```python
from build123d import *

# Parameters (mm, degrees)
F0_W     = 39.6748
F0_H     = 39.6748
F0_R     = 17.4625
F0_R_2   = 16.8275
F1_DEPTH = 3.2004
F2_DEPTH = 20.066
F3_R     = 13.97
F4_DEPTH = 16.8656
F5_R     = 15.5
F6_DEPTH = 8.1026


with BuildPart() as f1:
    # F0 (on Front) → F1 (new body)
    with BuildSketch(Plane.XZ):
        Rectangle(F0_W, F0_H)
        with BuildLine():
            Line((-13.265674, -15.564284), (-14.252556, -16.518023))
            ThreePointArc((-14.252556, -16.518023), (-16.635155, -16.817997), (-16.716767, -14.417977))
            Line((-16.716767, -14.417977), (-15.697317, -13.421976))
            ThreePointArc((-15.697317, -13.421976), (-13.320738, -13.175603), (-13.265674, -15.564284))
        make_face(mode=Mode.SUBTRACT)
        with BuildLine():
            ThreePointArc((13.323525, -15.493634), (13.405137, -13.093613), (15.787736, -13.393587))
            Line((15.787736, -13.393587), (16.774618, -14.347326))
            ThreePointArc((16.774618, -14.347326), (16.719554, -16.736007), (14.342975, -16.489634))
            Line((14.342975, -16.489634), (13.323525, -15.493634))
        make_face(mode=Mode.SUBTRACT)
        with BuildLine():
            ThreePointArc((-16.716767, 14.417977), (-16.635155, 16.817997), (-14.252556, 16.518023))
            Line((-14.252556, 16.518023), (-13.265674, 15.564284))
            ThreePointArc((-13.265674, 15.564284), (-13.320738, 13.175603), (-15.697317, 13.421976))
            Line((-15.697317, 13.421976), (-16.716767, 14.417977))
        make_face(mode=Mode.SUBTRACT)
        Circle(F0_R, mode=Mode.SUBTRACT)
        with BuildLine():
            Line((16.774618, 14.347326), (15.787736, 13.393587))
            ThreePointArc((15.787736, 13.393587), (13.405137, 13.093613), (13.323525, 15.493634))
            Line((13.323525, 15.493634), (14.342975, 16.489634))
            ThreePointArc((14.342975, 16.489634), (16.719554, 16.736007), (16.774618, 14.347326))
        make_face(mode=Mode.SUBTRACT)
        Circle(F0_R)
        Circle(F0_R_2, mode=Mode.SUBTRACT)
        Circle(F0_R_2)
    extrude(amount=F1_DEPTH)

    # F0 (on Front) → F2 (join)
    with BuildSketch(Plane.XZ):
        Circle(F0_R)
        Circle(F0_R_2, mode=Mode.SUBTRACT)
    extrude(amount=F2_DEPTH)

    # F3 (on face) → F4 (join)
    with BuildSketch(Plane.XZ.offset(3.2004)):
        with BuildLine():
            ThreePointArc((1.5875, -15.157092), (11.323672, -10.19961), (15.24, 0))
            ThreePointArc((15.24, 0), (-10.19961, 11.323672), (-1.5875, -15.157092))
            Line((-1.5875, -15.157092), (1.5875, -15.157092))
        make_face()
        Circle(F3_R, mode=Mode.SUBTRACT)
        with BuildLine():
            ThreePointArc((1.5875, -15.157092), (0, -15.24), (-1.5875, -15.157092))
            Line((-1.5875, -15.157092), (-1.5875, -16.427092))
            Line((-1.5875, -16.427092), (1.5875, -16.427092))
            Line((1.5875, -16.427092), (1.5875, -15.157092))
        make_face()
        with BuildLine():
            Line((1.5875, -15.157092), (-1.5875, -15.157092))
            ThreePointArc((-1.5875, -15.157092), (0, -15.24), (1.5875, -15.157092))
        make_face()
    extrude(amount=F4_DEPTH)

    # F5 (on face) → F6 (join)
    with BuildSketch(Plane(origin=(0, 0, 0), x_dir=(-1, 0, 0), z_dir=(0, 1, 0))):
        Circle(F5_R)
    extrude(amount=F6_DEPTH)


solid = f1.part
```
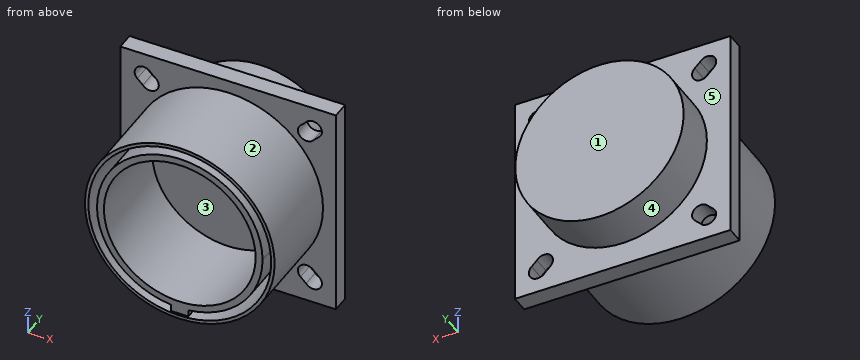
The listing builds one solid part. Answer for the finished solid, in the listing's coordinates (mm). Face numbers are marked on the shaded views. A direction names the side the tool comes from. Give positions to 0.01 mm unless a question says otherwise; leave off trailing zeros. Order: outer loops, then holes, each group sorted by start corner. A loop starts at its lowest first (then second) coordinate and runs counter-clockwise, first axis right, second up. Notation, with made-up numbers: M 25.25,81.25 L 45.25,81.25 A18 ccw 45.25,105.25 Z; hole C 73.25,41 d9. An arc over 180 degrees is marked long. Put each result on its own line as item: value. Start each with the question number.
Item 1: Which of the six approach directions +Z, -Z, +X, -X, +Y, -Y give full straight-line access (tool end or side, diameter ignored) to the marked faces 1 and 2?
Item 2: Find the intervals of material crossed by line 1 along X through (y, z) = (-6.75, -0.5); line 2 along X through (y, z) = (-1.75, -14.5); line 3 along X through (y, z) = (-6, -6.5), in increasing order.
Item 3: The part is cut by section C-C, the plane z = 6.5. Determine the outline of the cut face in (x, y), and give its area (3 significant figures).
Item 4: The part is cut by section B-B, the plane x = 8. Determine the outline of the cut face in (y, z), and give its area (3 significant figures).
Item 5: For a pull along X with two mould halves and no side action, classify the marked faces 3, 4 and 5 as +X half, -X half, draft (parallel to the pull), parting line (faces both ways), or undercut.
Item 6: The part is cut by section A-A, the plane y = -6. Determine the outline of the cut face in (x, z) (1 decimal), and give its area (3 significant figures).
Item 7: Flat-ended cylindrical pins translate along their axes: P1, Ø1, axis at y = -13.5, z = -16, coming from the -X side; P2, Ø2, axis at y = -13, z = 7.5, coming from the -X side; P3, Ø3, axis at x = 12, y = -8, coming from the -Z side. Find the tip coordinate at first contact, or state that the pin passes through.
Answer key:
1. face 1: +Z, -Z, +X, -X, +Y
1. face 2: -Y
2. line 1: x = -17.46 to -16.82, -15.23 to -13.96, 13.96 to 15.23, 16.82 to 17.46
2. line 2: x = -19.84 to -16.8, -12.77 to 12.84, 16.91 to 19.84
2. line 3: x = -16.21 to -15.52, -13.78 to -12.37, 12.37 to 13.78, 15.52 to 16.21
3. outline: M -19.84,-3.2 L -16.21,-3.2 L -16.21,-20.07 L -15.52,-20.07 L -15.52,-3.2 L -13.78,-3.2 L -13.78,-20.07 L -12.37,-20.07 L -12.37,-3.2 L 12.37,-3.2 L 12.37,-20.07 L 13.78,-20.07 L 13.78,-3.2 L 15.52,-3.2 L 15.52,-20.07 L 16.21,-20.07 L 16.21,-3.2 L 19.84,-3.2 L 19.84,0 L 14.07,0 L 14.07,8.1 L -14.07,8.1 L -14.07,0 L -19.84,0 Z
3. area: 426 mm²
4. outline: M -20.07,-15.52 L -3.2,-15.52 L -3.2,-19.84 L 0,-19.84 L 0,-13.28 L 8.1,-13.28 L 8.1,13.28 L 0,13.28 L 0,19.84 L -3.2,19.84 L -3.2,15.52 L -20.07,15.52 L -20.07,14.8 L -3.2,14.8 L -3.2,12.97 L -20.07,12.97 L -20.07,11.45 L -3.2,11.45 L -3.2,-11.45 L -20.07,-11.45 L -20.07,-12.97 L -3.2,-12.97 L -3.2,-14.8 L -20.07,-14.8 Z
4. area: 418 mm²
5. face 3: undercut
5. face 4: parting line
5. face 5: draft
6. outline: C 0,0 d34.9; M -1.6,-16.4 L 1.6,-16.4 L 1.6,-15.2 A15.2 ccw long -1.6,-15.2 Z; hole C 0,0 d33.7; hole C 0,0 d27.9
6. area: 189 mm²
7. P1: stops at x = -8.04
7. P2: stops at x = -16.21
7. P3: stops at z = -13.95
